Geometry: final body of the model. Coordinates: model frame, mm. A direction names the side the tool comes from. Coordinates: 2 decimals unless noted, no trailing zeros. Loops run counter-clockwise (first coordinate to the right, second up) from the corner with the lowest first, then second, coordinate; pieces in that order, holes last. Notation, with made-up numbers: (-3, 65.5) - (29, 65.5) arc R6 cw to (29, 69.5) - close; hole circle Ø3 at (27.25, 64). An arc over 180 degrees is marked (long way). Put each result on its own line as item: value. Start each with the question number.
1) Reachability of faces 1 (the cylindrical face through (9.673, 51.727, -14.705)), 2 (the flat face through (21, 49, 0)), 3 (the flat face through (23, 60.8, 0)) from +Z, -Z, +X, -X, +Y, -Y: full face, straight path, thin tool, end or side. Return the list, or none.
2) Section C-C on y = 54.9. Output: boundary loops of the cut face in (x, z).
3) Section B-B on z = -14. Count the separate pieces of the cut face and the enclosed holes in it, and give its area (3 significant figures).
4) Contact query for flat-ended pins moving along their axis: pin 1 Ø2.5 at (x, z) = (3.5, 6) entering from -Y; pin 2 Ø6.5 at (x, z) = (20.5, -12) entering from -Y; pin 3 Ø1.5 at (x, z) = (14.5, 15.5) entering from +Y; pin 4 Ø7.5 at (y, z) = (54.9, -14) entering from -X. Output: stop coordinate, or through.
5) Draft query along Y for faces 4 (the cylindrical face through (0.6, 70.43, 26.48)), 5 (the flat face through (9, 43, 28)), 6 (the flat face through (7, 22.5, 0)). Return one class per face: +Y half, -Y half, draft (parallel to the pull), parting line (faces both ways), or undercut.
6) Material intervals for line 1 along Z through (x, y) = (8.5, 54.9); line 2 along Y through (x, z) = (23.5, -14); line 3 along Y through (x, z) = (5, -14), sorted ascending. Write a range as from..to.
7) Section D-D on y = 31.5. Output: boundary loops of the cut face in (x, z).
8) Section A-A on x = 28. Output: boundary loops of the cut face in (y, z), and give its area (3 significant figures).
```python
from build123d import *

# Parameters (mm, degrees)
BOSS_EXTRUDE1_DEPTH                                 = 28
CBORE_FOR_M3_HEX_SOCKET_HEAD_CAP_SCREW1_D           = 3.4
CBORE_FOR_M3_HEX_SOCKET_HEAD_CAP_SCREW1_CBORE_D     = 6.5
CBORE_FOR_M3_HEX_SOCKET_HEAD_CAP_SCREW1_CBORE_DEPTH = 18.4
SKETCH5_W                                           = 3
SKETCH5_H                                           = 10.2
BOSS_EXTRUDE3_DEPTH                                 = 32
FILLET1_R                                           = 15
CUT_SWEEP1_START                                    = 17.5
CUT_SWEEP1_DEPTH                                    = 5
FILLET2_R                                           = 2


# Read off the part's stored shape, not the designer's step: Cut-Sweep1
with BuildPart() as part:
    # Sketch1 → Boss-Extrude1 (new, symmetric)
    with BuildSketch(Plane.XY):
        Polygon((0, 0), (0, 60.8), (32, 60.8), (32, 49), (10, 49), (10, 0), align=None)
    extrude(amount=BOSS_EXTRUDE1_DEPTH, both=True)

    # CBORE for M3 Hex Socket Head Cap Screw1 (through all)
    with Locations(Plane.ZY):
        with Locations((14, 54.9), (-14, 54.9)):
            CounterBoreHole(CBORE_FOR_M3_HEX_SOCKET_HEAD_CAP_SCREW1_D / 2, CBORE_FOR_M3_HEX_SOCKET_HEAD_CAP_SCREW1_CBORE_D / 2, CBORE_FOR_M3_HEX_SOCKET_HEAD_CAP_SCREW1_CBORE_DEPTH)

    # Sketch5 → Boss-Extrude3 (add)
    with BuildSketch(Plane(origin=(32, 0, 0), x_dir=(0, 0, -1), z_dir=(1, 0, 0))):
        with Locations((-26.5, 65.9)):
            Rectangle(SKETCH5_W, SKETCH5_H)
        with Locations((26.5, 65.9)):
            Rectangle(SKETCH5_W, SKETCH5_H)
    extrude(amount=-BOSS_EXTRUDE3_DEPTH)

    # Fillet1
    # the kernel refuses this fillet: 15 mm, written as the material it takes off along each edge
    with BuildSketch(Plane(origin=(0, 60.8, 25), x_dir=(0, -1, 0), z_dir=(0, 0, -1))) as fillet1_piece_1:
        with BuildLine():
            CenterArc((FILLET1_R, -FILLET1_R), FILLET1_R, 90, 90)
            Line((0, -FILLET1_R), (0, 0))
            Line((0, 0), (FILLET1_R, 0))
        make_face()
    extrude(amount=50, mode=Mode.SUBTRACT)

    # Cut-Sweep1 outline → Cut-Sweep1 (cut)
    with BuildSketch(Plane(origin=(0, 0, 0), x_dir=(1, 0, 0), z_dir=(0, 1, 0)).offset(CUT_SWEEP1_START)):
        with BuildLine():
            add(Edge.make_bspline(
                [(0, 21.25), (0.24543691, 21.25), (0.503005998, 21.185067302), (1.142972539, 20.803030792), (1.513644961, 20.479106412), (2.661593441, 19.052618916), (3.454291906, 17.504082361), (4.780601567, 13.525153377), (5.323721278, 11.098345132), (6.057965891, 5.780475225), (6.25, 2.890701574), (6.25, -2.890701574), (6.057965891, -5.780475225), (5.323721278, -11.098345132), (4.780601567, -13.525153377), (3.454291906, -17.504082361), (2.661593441, -19.052618916), (1.513644961, -20.479106412), (1.142972539, -20.803030792), (0.503005998, -21.185067302), (0.24543691, -21.25), (0, -21.25)],
                knots=[0.75, 0.75, 0.75, 0.75, 0.78125, 0.78125, 0.8125, 0.8125, 0.875, 0.875, 0.9375, 0.9375, 1, 1, 1.0625, 1.0625, 1.125, 1.125, 1.1875, 1.1875, 1.21875, 1.21875, 1.25, 1.25, 1.25, 1.25], degree=3))
            Line((0, -21.25), (0, -23.75))
            add(Edge.make_bspline(
                [(0, -23.75), (0.736310661, -23.75), (1.461325008, -23.524563287), (2.747539499, -22.756740545), (3.319589998, -22.222568191), (4.892691098, -20.267768767), (5.763908978, -18.480925296), (7.214400985, -14.129449273), (7.783074584, -11.564508722), (8.551624223, -5.998179833), (8.75, -2.999784652), (8.75, 2.999784652), (8.551624223, 5.998179833), (7.783074584, 11.564508722), (7.214400985, 14.129449273), (5.763908978, 18.480925296), (4.892691098, 20.267768767), (3.319589998, 22.222568191), (2.747539499, 22.756740545), (1.461325008, 23.524563287), (0.736310661, 23.75), (0, 23.75)],
                knots=[0, 0, 0, 0, 0.03125, 0.03125, 0.0625, 0.0625, 0.125, 0.125, 0.1875, 0.1875, 0.25, 0.25, 0.3125, 0.3125, 0.375, 0.375, 0.4375, 0.4375, 0.46875, 0.46875, 0.5, 0.5, 0.5, 0.5], degree=3))
            Line((0, 23.75), (0, 21.25))
        make_face()
    extrude(amount=CUT_SWEEP1_DEPTH, mode=Mode.SUBTRACT)

    # Fillet2
    fillet2_edges = [part.edges().sort_by_distance(p)[0] for p in [
        (0, 71, 26.5),
        (0, 71, -26.5),
    ]]
    fillet(fillet2_edges, radius=FILLET2_R)


solid = part.part
```
Answer block:
1. face 1: -X
1. face 2: +Z, -Z, +X, -Y
1. face 3: +X, -X, +Y
2. outline: (0, -28) - (32, -28) - (32, -15.7) - (18.4, -15.7) - (18.4, -17.25) - (3.08, -17.25) - (3.08, -25) - (0, -25) - close; (0, 25) - (3.08, 25) - (3.08, 17.25) - (18.4, 17.25) - (18.4, 15.7) - (32, 15.7) - (32, 28) - (0, 28) - close; (3.08, -10.75) - (18.4, -10.75) - (18.4, -12.3) - (32, -12.3) - (32, 12.3) - (18.4, 12.3) - (18.4, 10.75) - (3.08, 10.75) - close
3. separate pieces: 2
3. enclosed holes: 1
3. area: 662 mm²
4. pin 1: stops at y = 0
4. pin 2: stops at y = 49
4. pin 3: stops at y = 60.8
4. pin 4: stops at x = 0.99
5. face 4: +Y half
5. face 5: draft
5. face 6: undercut
6. line 1: z = -28..-17.25, -10.75..10.75, 17.25..28
6. line 2: y = 49..53.2, 56.6..60.8
6. line 3: y = 0..17.5, 22.5..51.65
7. outline: (0, -28) - (10, -28) - (10, 28) - (0, 28) - close
8. outline: (49, -28) - (71, -28) - (71, -25) - (60.8, -25) - (60.8, 25) - (71, 25) - (71, 28) - (49, 28) - close; hole circle Ø3.4 at (54.9, -14); hole circle Ø3.4 at (54.9, 14)
8. area: 704 mm²
